Job drawing, mm, ordinate dimensions from the low corner. One solid piece. A direction names the side the tool comes from. Give positions to 0.01 mm unless a question says otherwise; leave off trailing zeros. Loops run counter-clockwise (first coordinate to the right, second up) from the corner with the lowest first, then second, coordinate; pieces in that order, holes last. Notation, with made-up numbers: M 16,7.25 L 33,7.25 A19 cw 33,25.25 Z; hole C 9,81.25 d7. An arc over 180 degrees is marked long. Answer as CSV lines item,"result".
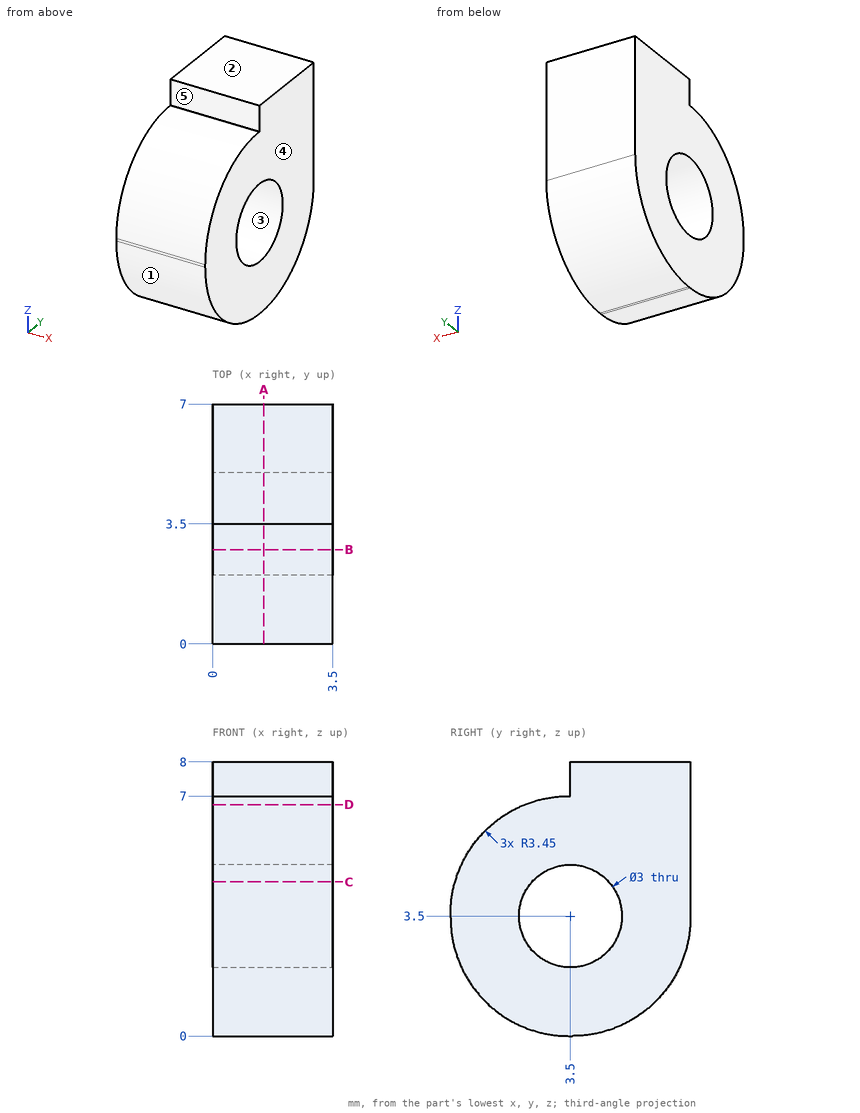
1) Band-saw the part on B-B on y = 2.75. Give the cut face in (x, z), and give its area (3 significant figures).
Answer below:
outline,"M 0,0.07 L 3.5,0.07 L 3.5,2.2 L 0,2.2 Z; M 0,4.8 L 3.5,4.8 L 3.5,6.93 L 0,6.93 Z"
area,"14.9 mm^2"
2) Band-saw the part on D-D on z = 6.75. Give the cut face in (x, y), and give its area (3 significant figures).
Answer below:
outline,"M 0,2.16 L 3.5,2.16 L 3.5,7 L 0,7 Z"
area,"16.9 mm^2"
3) Band-saw the part on C-C on z = 4.5. Give the cut face in (x, y).
Answer below:
outline,"M 0,0.13 L 3.5,0.13 L 3.5,2.38 L 0,2.38 Z; M 0,4.62 L 3.5,4.62 L 3.5,7 L 0,7 Z"
4) Which spindle directions (+Z, -Z, +X, -X, +Y, -Y) get a long thin tool onto all of the face, cutting with end or side? Do the marked faces 4 and 5. Say none if no direction does.
Answer below:
face 4,"+Z, -Z, +X, +Y, -Y"
face 5,"+Z, +X, -X, -Y"
5) Drill centre lines: line 1 (Y direction, x = 1.55, z = 3.5); line 2 (Y direction, x = 1.55, z = 7.5); line 3 (Z direction, x = 2.75, y = 2.75). Where is each one in solid material? Low to high. Write a range as from..to.
Answer below:
line 1,"y = 0..2, 5..7"
line 2,"y = 3.5..7"
line 3,"z = 0.07..2.2, 4.8..6.93"
6) Band-saw the part on A-A on x = 1.5. Give the cut face in (y, z).
Answer below:
outline,"M 0,3.45 A3.45 ccw 3.45,0 L 3.55,0 A3.45 ccw 7,3.45 L 7,8 L 3.5,8 L 3.5,7 L 3.45,7 A3.45 ccw 0,3.55 Z; hole C 3.5,3.5 d3"
7) Flat gauge pins, fed straight in: pin 1 (2.5 mm diameter, centred on y = 3.5, z = 3.5, fed in from -X); pin 2 (0.5 mm diameter, centred on x = 1.5, z = 7.5, fed in from -Y). Where does each tip first touch, or does it go through?
Answer below:
pin 1,"passes through"
pin 2,"stops at y = 3.5"
8) Mould opens along Z. For the marked faces 1, 2 and 3 say: +Z half, -Z half, draft (parallel to the pull), parting line (faces both ways), or undercut.
Answer below:
face 1,"-Z half"
face 2,"+Z half"
face 3,"undercut"
